Input: dimensioned drawing with shaded views. Units: mm. Origin: part minimum x, y, z. Coordinates: 2 decimals unless noted, no trailing zeros. Write each loop counter-clockwise with the first axis right and the second up, starting at its lowest first coordinate (ties: lowest second). Pieces come first, ordered by that corner, then holes. Notation, with made-up numbers: M 55.25,40.25 L 76.25,40.25 A21 ccw 76.25,77.25 Z; hole C 24.25,34.5 d6. An arc over 180 degrees is marked long. Use one line per item in the form item = value.
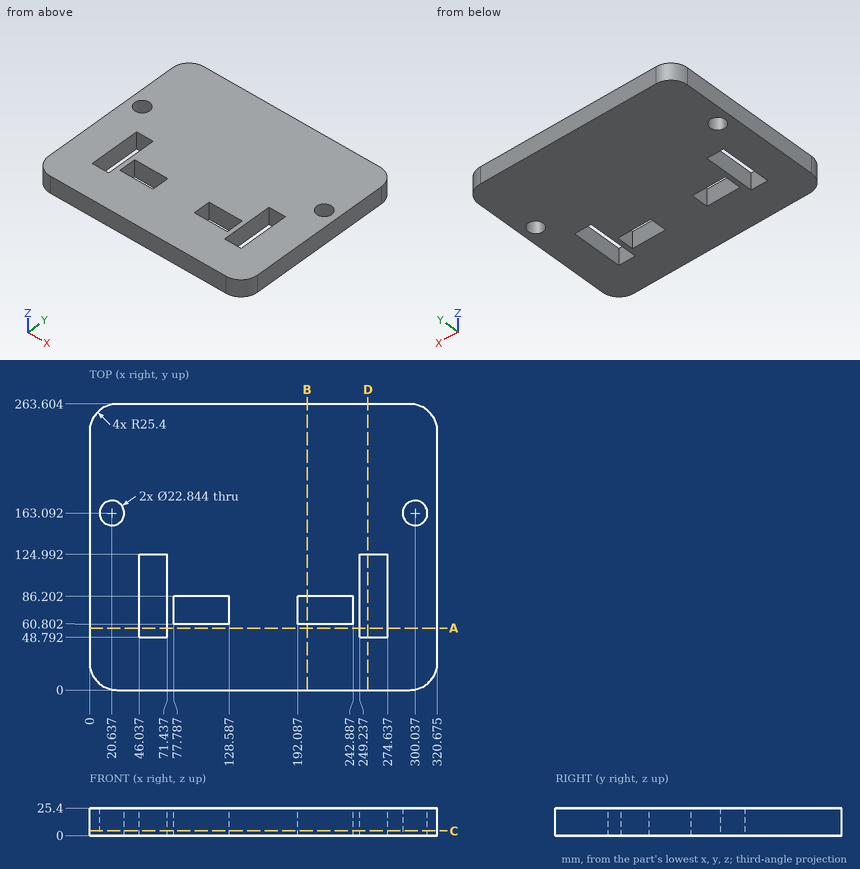
(1) Section query A-A on y = 57. Return the cut outline in (x, z) (1 decimal).
Computed:
outline = M 0,0 L 46,0 L 46,25.4 L 0,25.4 Z; M 71.4,0 L 249.2,0 L 249.2,25.4 L 71.4,25.4 Z; M 274.6,0 L 320.7,0 L 320.7,25.4 L 274.6,25.4 Z
(2) Section query D-D on x = 256.5. Return the cut outline in (y, z).
Computed:
outline = M 0,0 L 48.79,0 L 48.79,25.4 L 0,25.4 Z; M 124.99,0 L 263.6,0 L 263.6,25.4 L 124.99,25.4 Z
(3) Section query B-B on x = 200.5. Return the cut outline in (y, z), plus the area to 3 significant figures.
Computed:
outline = M 0,0 L 60.8,0 L 60.8,25.4 L 0,25.4 Z; M 86.2,0 L 263.6,0 L 263.6,25.4 L 86.2,25.4 Z
area = 6,050 mm^2
(4) Section query C-C on z = 4.25. Return the cut outline in (x, y) (1 decimal), plus the area to 3 significant figures.
Computed:
outline = M 0,25.4 A25.4 ccw 25.4,0 L 295.3,0 A25.4 ccw 320.7,25.4 L 320.7,238.2 A25.4 ccw 295.3,263.6 L 25.4,263.6 A25.4 ccw 0,238.2 Z; hole C 20.6,163.1 d22.8; hole M 46,48.8 L 71.4,48.8 L 71.4,125 L 46,125 Z; hole M 77.8,60.8 L 128.6,60.8 L 128.6,86.2 L 77.8,86.2 Z; hole M 192.1,60.8 L 242.9,60.8 L 242.9,86.2 L 192.1,86.2 Z; hole M 249.2,48.8 L 274.6,48.8 L 274.6,125 L 249.2,125 Z; hole C 300,163.1 d22.8
area = 76,700 mm^2
(5) Line query: probe 1 along X at (y, z) = (51.5, 5.5) (1 decimal); probe 2 along Y at (x, z) = (273, 2.5); probe 3 along Y at (x, z) = (98.5, 2.75). Output: solid intervals per line, ascending.
Computed:
probe_1 = 0 to 46, 71.4 to 249.2, 274.6 to 320.7
probe_2 = 0 to 48.79, 124.99 to 263.6
probe_3 = 0 to 60.8, 86.2 to 263.6
